```python
from build123d import *

# Parameters (mm, degrees)
SKETCH_1_W             = 150
SKETCH_1_H             = 93
EXTRUDE_1_DEPTH        = 90
FILLET_1_R             = 5
SHELL_1_T              = -4
EXTRUDE_3_DEPTH        = 10
FILLET_2_R             = 0.5
FILLET_2_OF_MIRROR_1_R = 0.5


with BuildPart() as part:
    # 草圖1 → 填料-伸長1 (new body)
    with BuildSketch(Plane(origin=(0, 0, 0), x_dir=(1, 0, 0), z_dir=(0, 1, 0))):
        Rectangle(SKETCH_1_W, SKETCH_1_H)
    extrude(amount=EXTRUDE_1_DEPTH)

    # 圓角1
    fillet_1_edges = [part.edges().sort_by_distance(p)[0] for p in [
        (0, 0, 46.5),
        (0, 0, -46.5),
    ]]
    fillet(fillet_1_edges, radius=FILLET_1_R)

    # 薄殼1
    shell_1_openings = [part.faces().sort_by_distance(p)[0] for p in [
        (0, 90, 0),
        (-75, 45.056329123, 0),
        (75, 45.056329123, 0),
    ]]
    offset(amount=SHELL_1_T, openings=shell_1_openings, kind=Kind.INTERSECTION)

    # 草圖2 → 填料-伸長3 (add)
    with BuildSketch(Plane(origin=(75, 0, 0), x_dir=(0, 0, -1), z_dir=(1, 0, 0))):
        Polygon((42.5, 59.7), (44.7, 61.9), (44.7, 28.1), (42.5, 30.3), align=None)
        Polygon((14.7, 4), (16.9, 1.8), (-16.9, 1.8), (-14.7, 4), align=None)
        Polygon((-42.5, 59.7), (-42.5, 30.3), (-44.7, 28.1), (-44.7, 61.9), align=None)
    extrude_3 = extrude(amount=EXTRUDE_3_DEPTH)

    # 圓角2
    fillet_2_edges = [part.edges().sort_by_distance(p)[0] for p in [
        (80, 59.7, -42.5),
        (80, 30.3, -42.5),
        (80, 28.1, -44.7),
        (80, 61.9, -44.7),
        (80, 4, -14.7),
        (80, 4, 14.7),
        (80, 1.8, 16.9),
        (80, 1.8, -16.9),
        (80, 61.9, 44.7),
        (80, 28.1, 44.7),
        (80, 30.3, 42.5),
        (80, 59.7, 42.5),
    ]]
    fillet(fillet_2_edges, radius=FILLET_2_R)

    # 鏡射1: 填料-伸長3 across plane
    add(extrude_3.mirror(Plane(origin=(0, 0, 0), x_dir=(0, 0, 1), z_dir=(1, 0, 0))))

    # 圓角2 of 鏡射1
    fillet_2_of_mirror_1_edges = [part.edges().sort_by_distance(p)[0] for p in [
        (-80, 59.7, -42.5),
        (-80, 30.3, -42.5),
        (-80, 28.1, -44.7),
        (-80, 61.9, -44.7),
        (-80, 4, -14.7),
        (-80, 4, 14.7),
        (-80, 1.8, 16.9),
        (-80, 1.8, -16.9),
        (-80, 61.9, 44.7),
        (-80, 28.1, 44.7),
        (-80, 30.3, 42.5),
        (-80, 59.7, 42.5),
    ]]
    fillet(fillet_2_of_mirror_1_edges, radius=FILLET_2_OF_MIRROR_1_R)


solid = part.part
```
Read the model definition and answer for the solid it produces. Units are mm, in the model's axes. A direction names the side the tool comes from. Round coordinates to 2 decimals unless told otherwise and drop trailing zeros. Write each loop counter-clockwise with the first axis right and the second up, starting at its lowest first coordinate (ties: lowest second). Pieces come first, ordered by that corner, then holes. Notation, with made-up numbers: (24, 62) - (43, 62) arc R16 ccw to (43, 85) - close; hole circle Ø3 at (62, 76.5). An arc over 180 degrees is marked (long way). One line per item, written item: value.
Q1. Which of the six approach directions +Z, -Z, +X, -X, +Y, -Y give full straight-line access (tool end or side, diameter ignored) to faces 5 (the flat face through (80, 1.8, 0)), 6 (the flat face through (-80, 45, 44.7)), 7 (the flat face through (-1, 4, -1))?
The answers:
face 5: +Z, -Z, +X, -Y
face 6: +Z, -X, +Y, -Y
face 7: +X, -X, +Y
Q2. Straight lines are drawn through the part: line 1 (Z direction, x = -6, y = 69); line 2 (Y direction, x = 39, z = -10.5); line 3 (Z direction, x = -76, y = 42). For each, find the intervals that lie inside material, in ascending order. Write a range as from..to.
The answers:
line 1: z = -46.5..-42.5, 42.5..46.5
line 2: y = 0..4
line 3: z = -44.7..-42.5, 42.5..44.7
Q3. For a pull along Z with two mould halves and no side action, classify faces 1 (the flat face through (-1, 47, 42.5)), 2 (the flat face through (-1, 47, 46.5)), 3 (the flat face through (-80, 1.8, 0)), 4 (the flat face through (80, 45, -44.7)) as pulls with the +Z half, pulls with the -Z half, needs draft (parallel to the pull), parting line crosses it, or undercut.
The answers:
face 1: undercut
face 2: pulls with the +Z half
face 3: needs draft
face 4: pulls with the -Z half
Q4. Find section C-C (x = -14). Determine the outline of the cut face in (y, z).
The answers:
outline: (0, -41.5) arc R5 ccw to (5, -46.5) - (90, -46.5) - (90, -42.5) - (5, -42.5) arc R1 cw to (4, -41.5) - (4, 41.5) arc R1 cw to (5, 42.5) - (90, 42.5) - (90, 46.5) - (5, 46.5) arc R5 ccw to (0, 41.5) - close
Q5. Find section B-B (z = -12). Determine the outline of the cut face in (x, y), and give its area (3 significant figures).
The answers:
outline: (-85, 1.8) - (-75, 1.8) - (-75, 0) - (75, 0) - (75, 1.8) - (85, 1.8) - (85, 4) - (-85, 4) - close
area: 644 mm2
Q6. Find section D-D (y = 84). Determine the outline of the cut face in (x, z), and give its area (3 significant figures).
The answers:
outline: (-75, -46.5) - (75, -46.5) - (75, -42.5) - (-75, -42.5) - close; (-75, 42.5) - (75, 42.5) - (75, 46.5) - (-75, 46.5) - close
area: 1,200 mm2
Q7. Each of these flat-tipped pins is pushed along its axis until it touches: P1, Ø8, axis at x = -78.5, y = 52, coming from the +Z side; P2, Ø3, axis at x = 82.5, z = -8, coming from the -Y side; P3, Ø2, axis at x = 43, z = -34, coming from the +Y side; P4, Ø5, axis at x = 79, y = 52, coming from the -Z side. Where does it stop, or does it pass through?
The answers:
P1: stops at z = 46.5
P2: stops at y = 1.8
P3: stops at y = 4
P4: stops at z = -44.7
Q8. Find section A-A (y = 48). Determine the outline of the cut face in (x, z).
The answers:
outline: (-85, -44.7) - (-75, -44.7) - (-75, -46.5) - (75, -46.5) - (75, -44.7) - (85, -44.7) - (85, -42.5) - (-85, -42.5) - close; (-85, 42.5) - (85, 42.5) - (85, 44.7) - (75, 44.7) - (75, 46.5) - (-75, 46.5) - (-75, 44.7) - (-85, 44.7) - close
